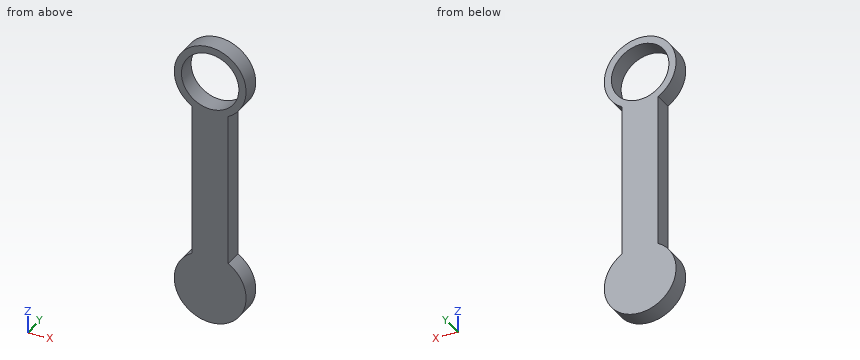
Autodesk Fusion 360 part; units mm, degrees
sketch "Boceto1" plane through (0, 0, 0) normal (0, 1, 0) x (1, 0, 0)
  circle A0 centre (0, 0) radius 8
  circle A1 centre (0, 0) radius 10
  line L0 (0, 0) -> (0, 70)
  line L1 (0, 70) -> (0, 60)
  circle A2 centre (0, 60) radius 10
  line L2 (0, 0) -> (-5, 0)
  line L3 (-5, 0) -> (-5, 51.3397)
  line L4 (0, 0) -> (5, 0)
  line L5 (5, 0) -> (5, 51.3397)
  dimension "d1" = 16
  dimension "d2" = 70
extrude "Extruir1" add sketch "Boceto1" along normal blind 5 contours A0 A1 L3 L5 | A0 A1 L0 L5 | A0 A1 L0 L3 | A1 L0 A2 L5 | A1 L0 A2 L3 | L0 L1 A2 | L0 L1 A2
ref_plane "PlanoDeObra1" through (0, 2.5396, -70) normal (0, 0, -1) x (1, 0, 0)
Geometry check sheet. Reference: the model listing, model coordinates, mm. Coordinates: 2 decimals unless noted, no trailing zeros. Write each loop counter-clockwise with the first axis right and the second up, starting at its lowest first coordinate (ties: lowest second). Pieces come first, ordered by that corner, then holes. Notation, with made-up numbers: (68, 56) -> (98, 56) arc R19 cw to (98, 83) -> close; hole circle Ø3 at (-25, 43.25). An arc over 180 degrees is marked (long way). Use CSV: the item, a comma, the result in double quotes. Start each with the question number.
Item 1: Cross-section at B-B, the plane x = 5.75. Record the cut outline in (y, z), plus the area to 3 significant figures.
Item 2: Cross-section at C-C, the plane x = 0. Record the cut outline in (y, z).
Item 3: Depth check by flat-ended pin: pin 1 Ø2 at (y, z) = (2, -37.5) entering from -X; pin 2 Ø2 at (x, y) = (-1.5, 1.5) entering from -Z; pin 3 Ø2 at (x, y) = (-7.5, 2) entering from +Z; pin 4 Ø3 at (x, z) = (-7.5, -32.5) entering from -Y. Enter the tip coordinate at first touch or a pass-through.
Item 4: Thickness scan on line 1 (Z direction, x = 0, y = 2.2); line 2 (X direction, y = 1.1, z = 0); line 3 (Z direction, x = -7.25, y = 2.55). Record the ranges inside material, lowest first.
Item 5: Cross-section at A-A, the plane z = 0. Record the cut outline in (x, y).
Item 6: Cross-section at D-D, the plane y = 2. Record the cut outline in (x, z).
Answers:
1,outline,"(0, -68.18) -> (5, -68.18) -> (5, -51.82) -> (0, -51.82) -> close; (0, -8.18) -> (5, -8.18) -> (5, -5.56) -> (0, -5.56) -> close; (0, 5.56) -> (5, 5.56) -> (5, 8.18) -> (0, 8.18) -> close"
1,area,"108 mm^2"
2,outline,"(0, -70) -> (5, -70) -> (5, -8) -> (0, -8) -> close; (0, 8) -> (5, 8) -> (5, 10) -> (0, 10) -> close"
3,pin 1,"x = -5"
3,pin 2,"z = -69.99"
3,pin 3,"z = 7.6"
3,pin 4,"through"
4,line 1,"-70 to -8, 8 to 10"
4,line 2,"-10 to -8, 8 to 10"
4,line 3,"-66.89 to -53.11, -6.89 to -3.38, 3.38 to 6.89"
5,outline,"(-10, 0) -> (-8, 0) -> (-8, 5) -> (-10, 5) -> close; (8, 0) -> (10, 0) -> (10, 5) -> (8, 5) -> close"
6,outline,"(-5, -51.34) arc R10 ccw (long way) to (5, -51.34) -> (5, -8.66) arc R10 ccw (long way) to (-5, -8.66) -> close; hole circle Ø16 at (0, 0)"
